from build123d import *

# Parameters (mm, degrees)
SKETCH_1_R               = 25
EXTRUDE_1_DEPTH          = 14
SKETCH_3_R               = 1.5
CUT_EXTRUDE_1_DEPTH      = 2
HOLE_WIZARD_M4_1_D       = 3.3
PATTERN_CIRCULAR_1_COUNT = 4
SKETCH_5_R               = 10
CUT_EXTRUDE_2_DEPTH      = 3
SKETCH_6_R               = 5
CUT_EXTRUDE_3_DEPTH      = 38.027017163


with BuildPart() as part:
    # 草图1 → 凸台-拉伸1 (new body)
    with BuildSketch(Plane.XY):
        Circle(SKETCH_1_R)
    extrude(amount=EXTRUDE_1_DEPTH)

    # 草图2 → 切除-旋转1 (revolve, cut)
    with BuildSketch(Plane(origin=(0, 0, 0), x_dir=(0, 0, -1), z_dir=(1, 0, 0)), mode=Mode.PRIVATE) as cut_revolve_1_sk:
        Polygon((-14, 25), (-2.5, 25), (-14, 23), align=None)
    revolve(cut_revolve_1_sk.sketch.rotate(Axis((0, 0, 0), (0, 0, -1)), 90), axis=Axis((0, 0, 0), (0, 0, -1)), mode=Mode.SUBTRACT)

    # 草图3 → 切除-拉伸1 (cut)
    with BuildSketch(Plane.XY.offset(14)):
        with Locations((13.435028843, 13.435028843)):
            Circle(SKETCH_3_R)
    extrude(amount=-CUT_EXTRUDE_1_DEPTH, mode=Mode.SUBTRACT)

    # M4 螺纹孔1 (through all)
    with Locations(Plane(origin=(13.435028843, 13.435028843, 14), x_dir=(1, 0, 0), z_dir=(0, 0, 1))):
        with Locations((0, 0)):
            hole_wizard_m4_1 = Hole(HOLE_WIZARD_M4_1_D / 2)

    # 阵列(圆周)1: M4 螺纹孔1 ×4 about axis
    pattern_circular_1_axis = Axis((0, 0, 0), (0, 0, 1))
    for i in range(1, PATTERN_CIRCULAR_1_COUNT):
        add(hole_wizard_m4_1.rotate(pattern_circular_1_axis, i * 360 / PATTERN_CIRCULAR_1_COUNT), mode=Mode.SUBTRACT)

    # 草图5 → 切除-拉伸2 (cut)
    with BuildSketch(Plane.XY.offset(14)):
        Circle(SKETCH_5_R)
    extrude(amount=-CUT_EXTRUDE_2_DEPTH, mode=Mode.SUBTRACT)

    # 草图6 → 切除-拉伸3 (cut, through all)
    with BuildSketch(Plane.XY.offset(11)):
        Circle(SKETCH_6_R)
    extrude(amount=-CUT_EXTRUDE_3_DEPTH, mode=Mode.SUBTRACT)


solid = part.part
The model under review builds one solid part; all positions refer to its coordinate system, in mm. A direction names the side the tool comes from. Coordinates: 2 decimals unless noted, no trailing zeros. Loops run counter-clockwise (first coordinate to the right, second up) from the corner with the lowest first, then second, coordinate; pieces in that order, holes last.
(1) Consider section D-D, the plane z = 7.5. Give the boundary of the cut face in (x, y).
Determined:
outline: circle Ø48.26 at (0, 0); hole circle Ø3.3 at (-13.44, -13.44); hole circle Ø3.3 at (-13.44, 13.44); hole circle Ø10 at (0, 0); hole circle Ø3.3 at (13.44, -13.44); hole circle Ø3.3 at (13.44, 13.44)
(2) Consider section A-A, the plane y = 0. Give the boundary of the cut face in (x, z), plus the area to 3 significant figures.
Determined:
outline: (-25, 0) - (-5, 0) - (-5, 11) - (-10, 11) - (-10, 14) - (-23, 14) - (-25, 2.5) - close; (5, 0) - (25, 0) - (25, 2.5) - (23, 14) - (10, 14) - (10, 11) - (5, 11) - close
area: 507 mm2
(3) Insertion check: P1, Ø1, axis at y = -10, z = 12.5, coming from the +X side; P2, Ø2, axis at x = -16.5, z = 12.5, coming from the -Y side; P3, Ø16, axis at x = 0, y = 0, coming from the +Z side. Each pin has a flat end and moves straight along its axis. Give the tip position at first contact, or say it passes through.
Determined:
P1: stops at x = 21.25
P2: stops at y = -17.37
P3: stops at z = 11
(4) Draft analysis for pull direction Y (two halves, no side actions). For faces 3 (the cylindrical face through (23.846, 7.509, 1.232)), 4 (the cylindrical face through (-15.083, -13.508, 6.902)), 5 (the flat face through (-0.3, -5.2, 0)), state which applies: +Y half, -Y half, draft (parallel to the pull), parting line (faces both ways), or undercut.
Determined:
face 3: parting line
face 4: undercut
face 5: draft
(5) Tool access review of faces 1 (the cylindrical face through (-1.08, -4.88, 5.58)), 2 (the flat face through (-5, -2, 11)): name each direction out of +Z, -Z, +X, -X, +Y, -Y from which nothing blocks a thin tool from reaching the whole face with its end or side.
Determined:
face 1: +Z, -Z
face 2: +Z
(6) Wall thickness on L1, parallel to X at y = 14, z = 8.75; L2, parallel to X at y = -3.5, z = 4; L3, parallel to Z at x = 6, y = 1: over which ranges is each line inside the solid? List them lowest first.
Determined:
L1: x = -19.39 to -14.99, -11.88 to 11.88, 14.99 to 19.39
L2: x = -24.49 to -3.57, 3.57 to 24.49
L3: z = 0 to 11
(7) Consider section C-C, the plane z = 3.75. Give the boundary of the cut face in (x, y), plus the area to 3 significant figures.
Determined:
outline: circle Ø49.57 at (0, 0); hole circle Ø3.3 at (-13.44, -13.44); hole circle Ø3.3 at (-13.44, 13.44); hole circle Ø10 at (0, 0); hole circle Ø3.3 at (13.44, -13.44); hole circle Ø3.3 at (13.44, 13.44)
area: 1,820 mm2
